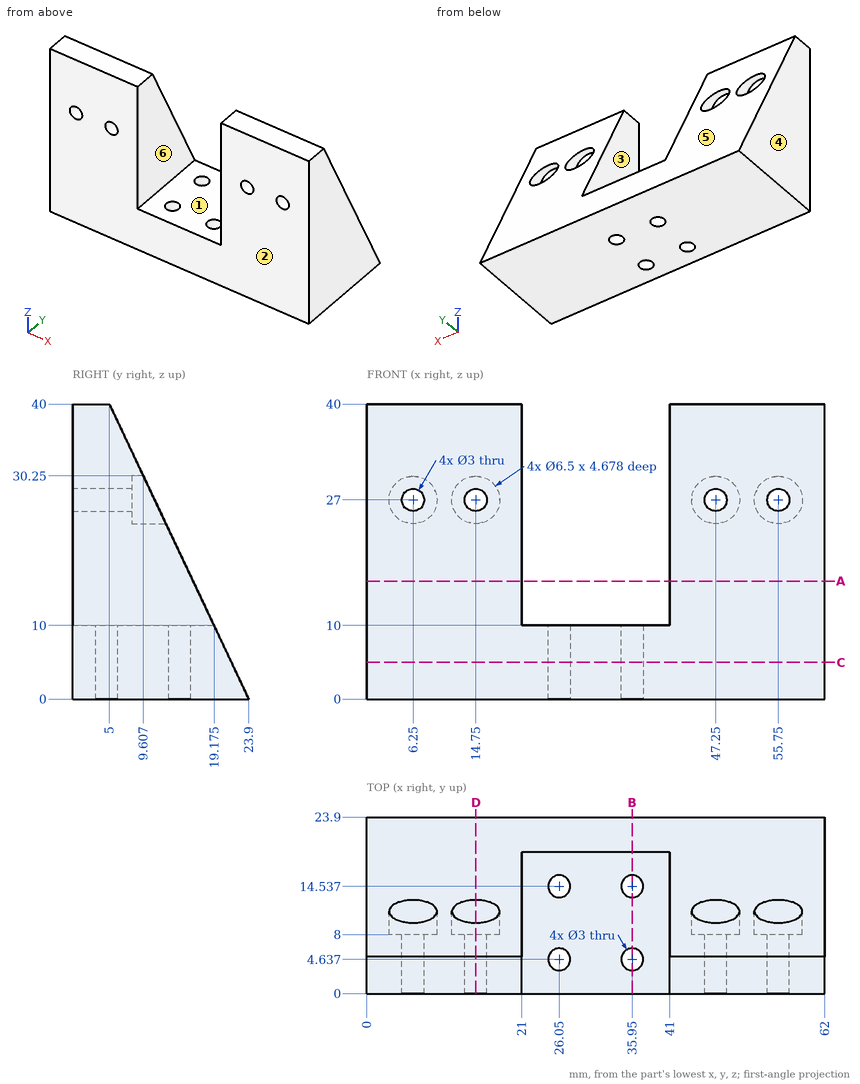
Geometry check sheet. Reference: drawing and pictorial views, mm from the part's lowest x, y, z. A direction names the side the tool comes from. Give positions to 0.01 mm unless a question says otherwise; leave off trailing zeros. Loops run counter-clockwise (first coordinate to the right, second up) from the corner with the lowest first, then second, coordinate; pieces in that order, holes last. Notation, with made-up numbers: (-29.5, 8.25) - (0.5, 8.25) arc R31 ccw to (0.5, 35.25) - close; hole circle Ø10 at (-34, 84.5). An arc over 180 degrees is marked (long way). Use CSV: the item, a comma, the result in double quotes. Start each with the question number.
Q1. Access from +Z, -Z, +X, -X, +Y, -Y to the whole of each face (thin tool, end or side, straight path). Record for the marked faces 5 and 6.
Q2. Scan lines: probe 1 along Y at (x, z) = (26.05, 3.75); probe 2 along X at (y, z) = (14.25, 15); probe 3 along Z at (x, y) = (31, 2.75). Record each from-to range of solid material in increasing order. Write a range as from..to.
Q3. Release check for a two-part mould opening along X. For the marked faces 1, 2, 3 and 4 record: +X half, -X half, draft (parallel to the pull), parting line (faces both ways), or undercut.
Q4. Section check B-B, the plane x = 35.95. Record the cut outline in (y, z) (1 decimal).
Q5. Section check A-A, the plane z = 16. Record the cut outline in (x, y), and give its area (3 significant figures).
Q6. Section check D-D, the plane x = 14.75. Record the cut outline in (y, z).
Q7. Section check C-C, the plane z = 5. Record the cut outline in (x, y), and give its area (3 significant figures).
Q8. Go/stop test with flat-tipped pins: pin 1 Ø3.5 at (x, z) = (6.25, 27) entering from +Y; pin 2 Ø12 at (x, z) = (55.5, 14.5) entering from -Y; pin 3 Ø3.5 at (x, y) = (26.05, 4.64) entering from +Z; pin 4 Ø5 at (x, z) = (15.5, 28) entering from +Y. Record where each tip stops, or that it passes through.
Findings below:
1,face 5,"+Z, +X, -X, +Y"
1,face 6,"+Z, +Y, -Y"
2,probe 1,"y = 0..3.14, 6.14..13.04, 16.04..22.13"
2,probe 2,"x = 0..21, 41..62"
2,probe 3,"z = 0..10"
3,face 1,"undercut"
3,face 2,"draft"
3,face 3,"undercut"
3,face 4,"-X half"
4,outline,"(0, 0) - (3.1, 0) - (3.1, 10) - (0, 10) - close; (6.1, 0) - (13, 0) - (13, 10) - (6.1, 10) - close; (16, 0) - (23.9, 0) - (19.2, 10) - (16, 10) - close"
5,outline,"(0, 0) - (21, 0) - (21, 16.34) - (0, 16.34) - close; (41, 0) - (62, 0) - (62, 16.34) - (41, 16.34) - close"
5,area,"686 mm^2"
6,outline,"(0, 0) - (23.9, 0) - (12.68, 23.75) - (8, 23.75) - (8, 25.5) - (0, 25.5) - close; (0, 28.5) - (8, 28.5) - (8, 30.25) - (9.61, 30.25) - (5, 40) - (0, 40) - close"
7,outline,"(0, 0) - (62, 0) - (62, 21.54) - (0, 21.54) - close; hole circle Ø3 at (26.05, 4.64); hole circle Ø3 at (26.05, 14.54); hole circle Ø3 at (35.95, 4.64); hole circle Ø3 at (35.95, 14.54)"
7,area,"1,310 mm^2"
8,pin 1,"stops at y = 8"
8,pin 2,"stops at y = 0"
8,pin 3,"stops at z = 10"
8,pin 4,"stops at y = 10.89"
